Design review of the part shown in the three views and the two pictorial views. Dimensions are in mm from the part's minimum x, y and z. A direction names the side the tool comes from. Coordinates: 2 decimals unless noted, no trailing zeros. Order: outer loops, then holes, each group sorted by start corner. A loop starts at its lowest first (then second) coordinate and runs counter-clockwise, first axis right, second up. Notation, with made-up numbers: (54.5, 19.5) -> (59.5, 19.5) arc R8 cw to (59.5, 23.5) -> close; hole circle Ø11 at (5, -4). An arc over 180 degrees is marked (long way). Write item = value, one per line. Start each with the question number.
1) Consider section C-C on z = 1.1. Give the boundary of the cut face in (x, y).
2) Machinability: for the marked faces 1 and 2, which of the approach directions +Z, -Z, +X, -X, +Y, -Y give a long, thin tool a straight path to every point of the face, cutting with its end or side? Answer none if there is none.
3) Consider section A-A on x = 5.95. Give the boundary of the cut face in (y, z).
4) Draft analysis for pull direction X (two halves, no side actions). For the marked faces 3, 4 and 5, state which applies: +X half, -X half, draft (parallel to the pull), parting line (faces both ways), or undercut.
5) Wall thickness on probe 1 along Y at (x, z) = (5.95, 3); probe 2 along Y at (x, z) = (5.95, 1); probe 3 along Z at (x, y) = (10.25, 7): over which ranges is each line inside the solid? List them lowest first. Write a range as [from, to].
6) Consider section D-D on x = 10.75. Give the boundary of the cut face in (y, z).
7) Insertion check: pin 1 Ø1.5 at (x, z) = (7.5, 0.5) entering from -Y; pin 2 Ø4.5 at (x, y) = (5.95, 5.95) entering from -Z. Each pin has a flat end and moves straight along its axis. Give the tip position at first contact, or say it passes through.
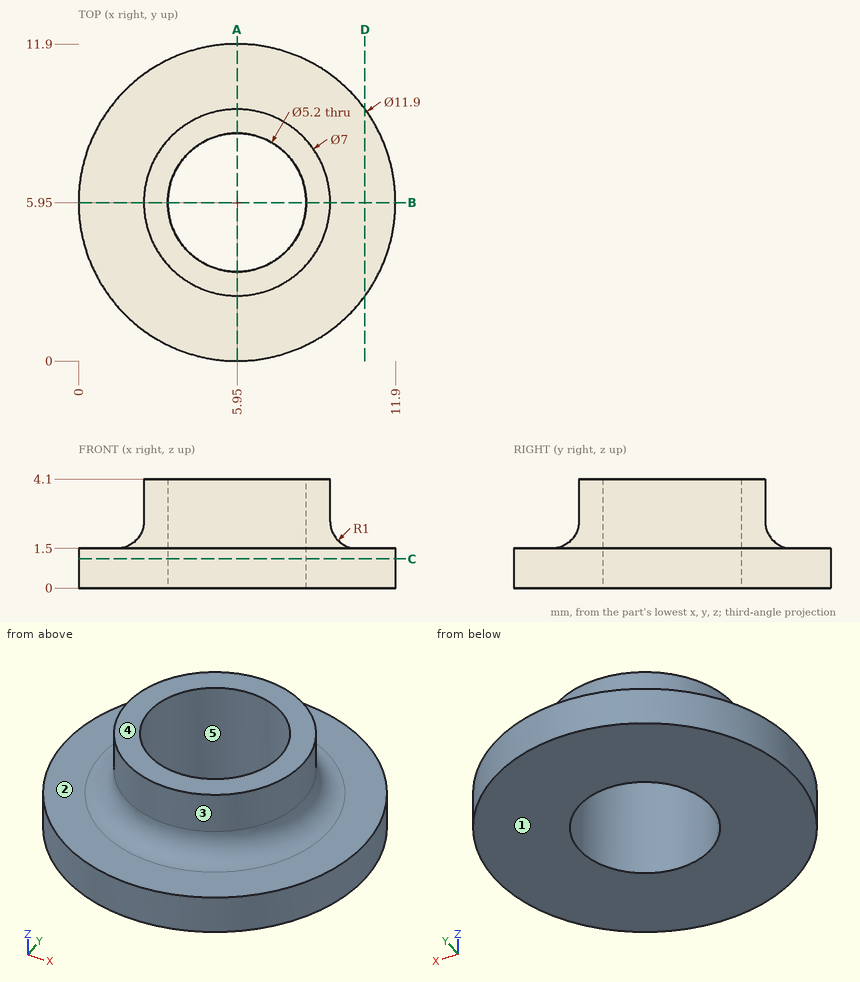
Answer sheet:
q1.outline = circle Ø11.9 at (5.95, 5.95); hole circle Ø5.2 at (5.95, 5.95)
q2.face_1 = -Z, +X, -X, +Y, -Y
q2.face_2 = +Z
q3.outline = (0, 0) -> (3.35, 0) -> (3.35, 4.1) -> (2.45, 4.1) -> (2.45, 2.5) arc R1 cw to (1.45, 1.5) -> (0, 1.5) -> close; (8.55, 0) -> (11.9, 0) -> (11.9, 1.5) -> (10.45, 1.5) arc R1 cw to (9.45, 2.5) -> (9.45, 4.1) -> (8.55, 4.1) -> close
q4.face_3 = parting line
q4.face_4 = draft
q4.face_5 = undercut
q5.probe_1 = [2.45, 3.35], [8.55, 9.45]
q5.probe_2 = [0, 3.35], [8.55, 11.9]
q5.probe_3 = [0, 1.5]
q6.outline = (2.43, 0) -> (9.47, 0) -> (9.47, 1.5) -> (2.43, 1.5) -> close
q7.pin_1 = 0.05
q7.pin_2 = through
